```python
from build123d import *

# Parameters (mm, degrees)
SKIZZE1_W                            = 57
SKIZZE1_H                            = 123
AUFSATZ_LINEAR_AUSTRAGEN1_DEPTH      = 2.5
SCHNITT_LINEAR_AUSTRAGEN1_DEPTH      = 84.889808678
SCHNITT_LINEAR_AUSTRAGEN2_DEPTH      = 68.828828679
SCHNITT_LINEAR_AUSTRAGEN3_DEPTH      = 70.726045338
SCHNITT_LINEAR_AUSTRAGEN3_DEPTH_BACK = 70.726045338
SCHNITT_LINEAR_AUSTRAGEN4_DEPTH      = 70.47454308
SCHNITT_LINEAR_AUSTRAGEN4_DEPTH_BACK = 70.47454308
SKIZZE9_W                            = 45.241474544
SKIZZE9_H                            = 11.280630507
AUFSATZ_LINEAR_AUSTRAGEN2_DEPTH      = 13
SCHNITT_LINEAR_AUSTRAGEN5_DEPTH      = 20
SKIZZE12_W                           = 36.023643564
SKIZZE12_H                           = 10.472363364
AUFSATZ_LINEAR_AUSTRAGEN3_DEPTH      = 5
SCHNITT_LINEAR_AUSTRAGEN6_DEPTH      = 12
SCHNITT_LINEAR_AUSTRAGEN8_DEPTH      = 0.5
SCHNITT_LINEAR_AUSTRAGEN8_DEPTH_BACK = 1.65
SKIZZE16_R                           = 3.1
SCHNITT_LINEAR_AUSTRAGEN9_DEPTH      = 1.15
SCHNITT_LINEAR_AUSTRAGEN9_DEPTH_BACK = 1
SKIZZE17_R                           = 3.1
SCHNITT_LINEAR_AUSTRAGEN10_DEPTH     = 10


with BuildPart() as part:
    # Skizze1 → Aufsatz-Linear austragen1 (new body)
    with BuildSketch(Plane(origin=(0, 0, 0), x_dir=(1, 0, 0), z_dir=(0, 1, 0))):
        Rectangle(SKIZZE1_W, SKIZZE1_H)
    extrude(amount=AUFSATZ_LINEAR_AUSTRAGEN1_DEPTH)

    # Skizze2 → Schnitt-Linear austragen1 (cut, through all)
    with BuildSketch(Plane(origin=(28.5, 0, 0), x_dir=(0, 0, -1), z_dir=(1, 0, 0))):
        Polygon((-61.5, 2.5), (-61.5, 0), (-60.968608596, 0), align=None)
    extrude(amount=-SCHNITT_LINEAR_AUSTRAGEN1_DEPTH, mode=Mode.SUBTRACT)

    # Skizze3 → Schnitt-Linear austragen2 (cut, through all)
    with BuildSketch(Plane(origin=(0, 2.5, 0), x_dir=(1, 0, 0), z_dir=(0, 1, 0))):
        Polygon((-28.5, -61.5), (-17.738894386, 61.5), (-28.5, 61.5), align=None)
        Polygon((28.5, -61.5), (17.738894386, 61.5), (28.5, 61.5), align=None)
    extrude(amount=-SCHNITT_LINEAR_AUSTRAGEN2_DEPTH, mode=Mode.SUBTRACT)

    # Skizze5 → Schnitt-Linear austragen3 (cut, two sides: drawn at the far end of the back side and taken through both)
    with BuildSketch(Plane(origin=(0.175618176, 0, 2.007324937), x_dir=(0, -1, 0), z_dir=(0.08715574274765484, 0, 0.9961946980917459)).offset(-SCHNITT_LINEAR_AUSTRAGEN3_DEPTH_BACK)):
        Polygon((0.008562414, 23.031470717), (-2.5, 23.031470717), (0, 21.995936811), align=None)
    extrude(amount=SCHNITT_LINEAR_AUSTRAGEN3_DEPTH + SCHNITT_LINEAR_AUSTRAGEN3_DEPTH_BACK, mode=Mode.SUBTRACT)

    # Skizze6 → Schnitt-Linear austragen4 (cut, two sides: drawn at the far end of the back side and taken through both)
    with BuildSketch(Plane(origin=(-0.152372814, 0, 1.741629235), x_dir=(0, 1, 0), z_dir=(-0.08715574274766175, 0, 0.9961946980917452)).offset(-SCHNITT_LINEAR_AUSTRAGEN4_DEPTH_BACK)):
        Polygon((2.5, 23.031470717), (0, 21.995936811), (0, 23.031470717), align=None)
    extrude(amount=SCHNITT_LINEAR_AUSTRAGEN4_DEPTH + SCHNITT_LINEAR_AUSTRAGEN4_DEPTH_BACK, mode=Mode.SUBTRACT)

    # Skizze9 → Aufsatz-Linear austragen2 (add)
    with BuildSketch(Plane.XZ):
        with Locations((0, 52.468608596)):
            Rectangle(SKIZZE9_W, SKIZZE9_H)
    extrude(amount=AUFSATZ_LINEAR_AUSTRAGEN2_DEPTH)

    # Skizze11 → Schnitt-Linear austragen5 (cut)
    with BuildSketch(Plane(origin=(0, 0, 46.828293342), x_dir=(-1, 0, 0), z_dir=(0, 0, -1))):
        Polygon((-22.620737272, -9.484039906), (0, 0), (22.620737272, -9.484039906), (22.620737272, -13), (-22.620737272, -13), align=None)
    extrude(amount=-SCHNITT_LINEAR_AUSTRAGEN5_DEPTH, mode=Mode.SUBTRACT)

    # Skizze12 → Aufsatz-Linear austragen3 (add)
    with BuildSketch(Plane.XZ):
        with Locations((0, -20.5)):
            Rectangle(SKIZZE12_W, SKIZZE12_H)
    extrude(amount=AUFSATZ_LINEAR_AUSTRAGEN3_DEPTH)

    # Skizze13 → Schnitt-Linear austragen6 (cut)
    with BuildSketch(Plane(origin=(0, 0, -25.736181682), x_dir=(-1, 0, 0), z_dir=(0, 0, -1))):
        Polygon((-18.011821782, -2.5), (-7.183132097, 0), (7.183132097, 0), (18.011821782, -2.5), (18.011821782, -5), (-18.011821782, -5), align=None)
    extrude(amount=-SCHNITT_LINEAR_AUSTRAGEN6_DEPTH, mode=Mode.SUBTRACT)

    # Skizze16 → Schnitt-Linear austragen8 (cut, two sides: drawn at the far end of the back side and taken through both)
    with BuildSketch(Plane.XZ.offset(-SCHNITT_LINEAR_AUSTRAGEN8_DEPTH_BACK)):
        with Locations(Location((12.59747694, -20.5, 0), (0, 0, 270))):
            Circle(SKIZZE16_R)
        with Locations(Location((-12.59747694, -20.5, 0), (0, 0, 270))):
            Circle(SKIZZE16_R)
    extrude(amount=SCHNITT_LINEAR_AUSTRAGEN8_DEPTH + SCHNITT_LINEAR_AUSTRAGEN8_DEPTH_BACK, mode=Mode.SUBTRACT)

    # Skizze17 → Schnitt-Linear austragen9 (cut, two sides: drawn at the far end of the back side and taken through both)
    with BuildSketch(Plane(origin=(0, -4.742019953, 0), x_dir=(1, 0, 0), z_dir=(0, 1, 0)).offset(-SCHNITT_LINEAR_AUSTRAGEN9_DEPTH_BACK)):
        with Locations(Location((-16.965552954, -52.468608596, 0), (0, 0, 270))):
            Circle(SKIZZE17_R)
        with Locations(Location((16.965552954, -52.468608596, 0), (0, 0, 270))):
            Circle(SKIZZE17_R)
    extrude(amount=SCHNITT_LINEAR_AUSTRAGEN9_DEPTH + SCHNITT_LINEAR_AUSTRAGEN9_DEPTH_BACK, mode=Mode.SUBTRACT)

    # Skizze18 → Schnitt-Linear austragen10 (cut)
    with BuildSketch(Plane(origin=(0, 2.5, 0), x_dir=(1, 0, 0), z_dir=(0, 1, 0))):
        with BuildLine():
            Line((-9.738894386, 61.5), (-9.738894386, 42.49))
            ThreePointArc((-9.738894386, 42.49), (-12.718555412, 35.29646194), (-19.912093472, 32.316800915))
            Line((-19.912093472, 32.316800915), (-20.292093472, 32.316800915))
            Line((-20.292093472, 32.316800915), (-17.738894386, 61.5))
            Line((-17.738894386, 61.5), (-9.738894386, 61.5))
        make_face()
    extrude(amount=-SCHNITT_LINEAR_AUSTRAGEN10_DEPTH, mode=Mode.SUBTRACT)


solid = part.part
```
CAD build for the part. Positions are in the model's coordinates, mm. A direction names the side the tool comes from. Coordinates: 2 decimals unless noted, no trailing zeros. Order: outer loops, then holes, each group sorted by start corner. A loop starts at its lowest first (then second) coordinate and runs counter-clockwise, first axis right, second up.
(1) Which spindle directions (+Z, -Z, +X, -X, +Y, -Y) get a long thin tool onto all of the face, cutting with end or side? Do faces 1 (the face through (13, 1.65, -20)), 2 (the face through (-11.152, -4.676, 52.39)), 3 (the face through (-22.621, -5, 52)), 4 (the face through (-12.522, -1.232, -20.573)), 5 (the face through (22.621, -5, 52)). Say none if no direction does.
Solution:
face 1: none
face 2: +Z, -Z, -Y
face 3: +Z, -Z, -X, -Y
face 4: -Z, -Y
face 5: +Z, -Z, +X, -Y
(2) Saw through at B-B, the plane x = 11.5. Write the cut outline in (y, z).
Solution:
outline: (-4.82, 46.83) - (0, 46.83) - (0, -15.26) - (-1, -15.26) - (-1, -25.74) - (0, -25.74) - (0, -61.5) - (2.5, -61.5) - (2.5, 61.5) - (0, 60.97) - (0, 58.11) - (-4.82, 58.11) - close; hole (-0.5, -23.4) - (1.65, -23.4) - (1.65, -17.6) - (-0.5, -17.6) - close
(3) Saw through at D-D, the plane x = 3. Write the cut outline in (y, z).
Solution:
outline: (-1.26, 46.83) - (0, 46.83) - (0, -61.5) - (2.5, -61.5) - (2.5, 61.5) - (0, 60.97) - (0, 58.11) - (-1.26, 58.11) - close
(4) Drill centre lines: L1, parallel to X at y = 1.2, z = -20.5; L2, parallel to X at y = 0.85, z = -20.5; L3, parallel to Y at x = -5.5, z = -36.5. Where is each one in solid material? Low to high.
Solution:
L1: x = -20.79 to -15.7, -9.5 to 9.5, 15.7 to 20.79
L2: x = -20.64 to -15.7, -9.5 to 9.5, 15.7 to 20.64
L3: y = 0 to 2.5
(5) Saw through at A-A, the plane z = -20.5. Write the cut outline in (x, y).
Solution:
outline: (-21.33, 2.5) - (-20.29, 0) - (-18.01, 0) - (-18.01, -2.5) - (-7.18, 0) - (7.18, 0) - (18.01, -2.5) - (18.01, 0) - (20.29, 0) - (21.33, 2.5) - close; hole (-15.7, -0.5) - (-9.5, -0.5) - (-9.5, 1.65) - (-15.7, 1.65) - close; hole (9.5, -0.5) - (15.7, -0.5) - (15.7, 1.65) - (9.5, 1.65) - close
(6) Saw through at C-C, the plane z = 48. Write the cut outline in (x, y), and give its area (3 significant figures).
Solution:
outline: (-27.32, 2.5) - (-26.28, 0) - (-22.62, 0) - (-22.62, -9.48) - (0, 0) - (22.62, -9.48) - (22.62, 0) - (26.28, 0) - (27.32, 2.5) - close
area: 349 mm2
(7) Pin check, flat tips, straight feed: pin 1 Ø6 at (x, y) = (-9, -6.5) entering from -Z; pin 2 Ø4.5 at (x, y) = (-11, -3) entering from -Z; pin 3 Ø4.5 at (y, z) = (-7, 51.5) entering from -X. Stop position of each tip, or through.
Solution:
pin 1: stops at z = 46.83
pin 2: stops at z = -25.74
pin 3: stops at x = -22.62
(8) Mould opens along Z. For faces 6 (the face through (15, -1, -25.736)), 7 (the face through (0.4, 1.23, 61.23)), 8 (the face through (12.673, -1.268, -20.573)), 9 (the face through (-18.153, -4.682, 55.332)) say: released by +Z, released by -Z, zero draft, split by the parting line, or undercut.
Solution:
face 6: released by -Z
face 7: released by +Z
face 8: zero draft
face 9: undercut
